Read the model definition and answer for the solid it produces. Units are mm, in the model's axes. A direction names the side the tool comes from. Give positions to 0.01 mm unless a question says otherwise; leave off trailing zeros. Write each loop counter-clockwise with the first axis right and the second up, starting at its lowest first coordinate (ties: lowest second). Pieces come first, ordered by that corner, then holes. Notation, with made-up numbers: (43.5, 64) -> (89.5, 64) arc R22 ccw to (89.5, 98) -> close; hole circle Ø8 at (32.5, 57). An arc over 180 degrees is marked (long way). Put each result on its own line as item: value. Start each with the question number.
from build123d import *

# Parameters (mm, degrees)
SKETCH1_W           = 9.144
SKETCH1_H           = 23.0378
BOSS_EXTRUDE1_DEPTH = 5.715


with BuildPart() as part:
    # Sketch1 → Boss-Extrude1 (new body)
    # profile 1 of 2: a face of its own
    with BuildSketch(Plane(origin=(0, 0, 0), x_dir=(1, 0, 0), z_dir=(0, 1, 0))):
        Polygon((38.4175, 110.49), (41.275, 110.49), (44.1325, 110.49), (44.1325, 0), (82.55, 0), (82.55, 241.3), (0, 241.3), (0, 0), (38.4175, 0), align=None)
        with Locations((25.146, 217.0811)):
            Rectangle(SKETCH1_W, SKETCH1_H, mode=Mode.SUBTRACT)
        with Locations((57.404, 217.0811)):
            Rectangle(SKETCH1_W, SKETCH1_H, mode=Mode.SUBTRACT)
    # profile 2 of 2: a face of its own
    with BuildSketch(Plane(origin=(0, 0, 0), x_dir=(1, 0, 0), z_dir=(0, 1, 0))):
        Polygon((38.4175, 110.49), (41.275, 110.49), (44.1325, 110.49), (44.1325, 0), (82.55, 0), (82.55, 241.3), (0, 241.3), (0, 0), (38.4175, 0), align=None)
        with Locations((25.146, 217.0811)):
            Rectangle(SKETCH1_W, SKETCH1_H, mode=Mode.SUBTRACT)
        with Locations((57.404, 217.0811)):
            Rectangle(SKETCH1_W, SKETCH1_H, mode=Mode.SUBTRACT)
    extrude(amount=BOSS_EXTRUDE1_DEPTH)


solid = part.part
1) A cutting plane is placed at B-B on x = 25. Give the vertices of the cut face in (y, z) (3 decimals).
2) This flat-tipped pin is pushed along its axis until it touches: pin 1 Ø3 at (x, y) = (42.5, 4) entering from +Z. Where does it stop, or does it pass through?
3) Straight lines are drawn through the part: line 1 (X direction, y = 1.8, z = -106); line 2 (X direction, y = 5.2, z = -213); line 3 (Z direction, x = 55.5, y = 2.1). For each, find the intervals that lie inside material, in ascending order. Write a range as [from, to].
4) A cutting plane is placed at C-C on y = 3. Give the vertices of the cut face in (x, z), and give its area (3 significant figures).
5) For faces 5 (the face through (57, 3, -228.6)), 6 (the face through (38.418, 3, -54)), 7 (the face through (41, 5.715, -122)), determine the directions among +Z, -Z, +X, -X, +Y, -Y from which every point of the face is accessible in a straight line to the end or side of a thin tool.
6) For a pull along X with two mould halves and no side action, classify faces 1 (the face through (63, 3, 0)), 2 (the face through (61.976, 3, -217)), 3 (the face through (82.55, 3, -119)), 4 (the face through (0, 3, -122)) as pulls with the +X half, pulls with the -X half, needs draft (parallel to the pull), parting line crosses it, or undercut.
7) A cutting plane is placed at D-D on x = 41. Give the vertices of the cut face in (y, z) (3 decimals).
Results found:
1. outline: (0, -241.3) -> (5.715, -241.3) -> (5.715, -228.6) -> (0, -228.6) -> close; (0, -205.562) -> (5.715, -205.562) -> (5.715, 0) -> (0, 0) -> close
2. pin 1: stops at z = -110.49
3. line 1: x = [0, 38.42], [44.13, 82.55]
3. line 2: x = [0, 20.57], [29.72, 52.83], [61.98, 82.55]
3. line 3: z = [-241.3, -228.6], [-205.56, 0]
4. outline: (0, -241.3) -> (82.55, -241.3) -> (82.55, 0) -> (44.13, 0) -> (44.13, -110.49) -> (38.42, -110.49) -> (38.42, 0) -> (0, 0) -> close; hole (20.57, -228.6) -> (29.72, -228.6) -> (29.72, -205.56) -> (20.57, -205.56) -> close; hole (52.83, -228.6) -> (61.98, -228.6) -> (61.98, -205.56) -> (52.83, -205.56) -> close
4. area: 18,900 mm²
5. face 5: +Y, -Y
5. face 6: +Z, +Y, -Y
5. face 7: +Z, -Z, +X, -X, +Y
6. face 1: needs draft
6. face 2: undercut
6. face 3: pulls with the +X half
6. face 4: pulls with the -X half
7. outline: (0, -241.3) -> (5.715, -241.3) -> (5.715, -110.49) -> (0, -110.49) -> close
